Here's how the part is built. I have some questions about the finished solid (model axes, mm). A direction names the side the tool comes from. Round coordinates to 2 decimals unless told otherwise and drop trailing zeros. Order: outer loops, then holes, each group sorted by start corner. A loop starts at its lowest first (then second) coordinate and runs counter-clockwise, first axis right, second up. Notation, with made-up numbers: (-12, -34.5) -> (-2, -34.5) arc R12 cw to (-2, -23.5) -> close; hole circle Ø6 at (86.5, -16.75). An arc over 180 degrees is marked (long way). Use a Markdown table: item, result. Add a question column.
Autodesk Inventor part; units mm, degrees
ref_plane "YZ Plane" through (0, 0, 0) normal (1, 0, 0) x (0, 1, 0)
ref_plane "XZ Plane" through (0, 0, 0) normal (0, 1, 0) x (-1, 0, 0)
ref_plane "XY Plane" through (0, 0, 0) normal (0, 0, 1) x (1, 0, 0)
sketch "Sketch1" plane through (0, 0, 0) normal (0, 0, 1) x (1, 0, 0)
  line L0 (0, 0) -> (525.78, 0)
  line L1 (0, 0) -> (0, 101.6)
  line L2 (0, 101.6) -> (262.89, 253.3796)
  line L3 (262.89, 253.3796) -> (525.78, 101.6)
  line L4 (525.78, 101.6) -> (525.78, 0)
  line L5 (262.89, 246.0473) -> (6.35, 97.9338)
  line L6 (6.35, 97.9338) -> (6.35, 6.35)
  line L7 (6.35, 6.35) -> (519.43, 6.35)
  line L8 (519.43, 6.35) -> (519.43, 97.9338)
  line L9 (519.43, 97.9338) -> (262.89, 246.0473)
  point P0 (262.89, 0)
  dimension "d0" = 525.78
  dimension "d1" = 101.6
  dimension "d2" = 120
  dimension "d3" = 6.35
extrude "Extrusion1" add sketch "Sketch1" along normal blind 355.6
sketch "Sketch2" plane through (0, 0, 355.6) normal (0, 0, 1) x (1, 0, 0)
  line L0 (262.89, 246.0473) -> (519.43, 97.9338)
  line L1 (519.43, 97.9338) -> (519.43, 6.35)
  line L2 (519.43, 6.35) -> (6.35, 6.35)
  line L3 (6.35, 6.35) -> (6.35, 97.9338)
  line L4 (6.35, 97.9338) -> (262.89, 246.0473)
  line L5 (0, 0) -> (525.78, 0)
  line L6 (525.78, 0) -> (525.78, 101.6)
  line L7 (525.78, 101.6) -> (262.89, 253.3796)
  line L8 (262.89, 253.3796) -> (0, 101.6)
  line L9 (0, 101.6) -> (0, 0)
  circle A0 centre (262.89, 121.3796) radius 60
  dimension "d6" = 120
  dimension "d7" = 132
extrude "Extrusion2" add sketch "Sketch2" along normal blind 6.35 contours L0 L1 L2 L3 L4 | L9 L8 L7 L6 L5
sketch "Sketch3" plane through (0, 0, 0) normal (0, -1, 0) x (1, 0, 0)
  line L0 (0, 0) -> (525.78, 0) construction
  line L1 (525.78, 0) -> (525.78, 88.9)
  line L2 (525.78, 88.9) -> (0, 88.9) construction
  line L3 (0, 88.9) -> (0, 0) construction
  line L4 (86.36, 21.95) -> (86.36, 66.95) construction
  circle A0 centre (86.36, 44.45) radius 2.3812
  circle A1 centre (86.36, 21.95) radius 2.3812
  circle A2 centre (86.36, 66.95) radius 2.3812
  line L5 (146.36, 49.45) -> (146.36, 29.45) construction
  line L6 (156.36, 66.95) -> (156.36, 21.95) construction
  line L7 (146.36, 29.45) -> (166.36, 29.45) construction
  line L8 (166.36, 49.45) -> (146.36, 49.45) construction
  line L9 (86.36, 66.95) -> (226.36, 66.95) construction
  line L10 (226.36, 21.95) -> (86.36, 21.95) construction
  line L11 (86.36, 44.45) -> (226.36, 44.45) construction
  line L12 (166.36, 29.45) -> (166.36, 49.45) construction
  line L13 (226.36, 66.95) -> (226.36, 21.95) construction
  circle A3 centre (226.36, 66.95) radius 2.3813
  circle A4 centre (226.36, 44.45) radius 2.3813
  circle A5 centre (226.36, 21.95) radius 2.3813
  circle A6 centre (156.36, 39.45) radius 10
  line L14 (0, 0) -> (0, 361.95)
  line L15 (525.78, 0) -> (525.78, 361.95)
  line L16 (0, 0) -> (525.78, 0)
  point P0 (0, 44.45)
  point P1 (146.36, 39.45)
  point P2 (166.36, 39.45)
  point P3 (262.89, 0)
  dimension "d10" = 45
  dimension "d11" = 140
  dimension "d12" = 4.7625
  dimension "d13" = 4.7625
  dimension "d14" = 4.7625
  dimension "d15" = 4.7625
  dimension "d16" = 4.7625
  dimension "d17" = 4.7625
  dimension "d18" = 60
  dimension "d19" = 7.5
  dimension "d20" = 20
  dimension "d21" = 20
  dimension "d22" = 86.36
  dimension "d23" = 88.9
extrude "Extrusion3" cut sketch "Sketch3" against normal blind 6.35
sketch "Sketch4" plane through (0, 0, 0) normal (0, -1, 0) x (1, 0, 0)
  line L0 (71.36, 0) -> (241.36, 0)
  line L1 (241.36, 0) -> (241.36, 85)
  line L2 (241.36, 85) -> (71.36, 85)
  line L3 (71.36, 85) -> (71.36, 0)
  line L4 (0, 0) -> (525.78, 0) construction
  circle A0 centre (156.36, 39.45) radius 10 construction
  point P0 (156.36, 85)
  dimension "d26" = 170
  dimension "d27" = 85
extrude "Extrusion4" [suppressed]
properties part number "CA01" material "ABS Plastic"
(1) On a 3-axis mill with a long thin cutter (end or side, diameter ignored), from which of +Z, -Z, +X, -X, +Y, -Y can I reach the whole of each face in a straight line? I mean faces 5 (the flat face through (129.605, 176.427, 178.441)), 6 (the flat face through (6.35, 53, 175)), 7 (the cylindrical face through (165.9, 3.13, 42.45)). Say none if no direction works.
(2) If we mould it in two halves opening along X, with no side actions, what happens to faces 1 (the flat face through (259, 48, 355.6)), 2 (the flat face through (525.78, 52, 178)), 3 (the flat face through (136.42, 173.03, 175.31)), 4 (the flat face through (0, 50, 178))? For each: pulls with the +X half, pulls with the -X half, needs draft (parallel to the pull), parting line crosses it, or undercut.
(3) I want a section at B-B on y = 75. List the corners of the cut face in (x, z) for me, and give its area (3 significant figures).
(4) I want a section at D-D on x = 436.5. List the corners of the cut face in (y, z) for me, and give its area (3 significant figures).
(5) I want a section at A-A on z = 326. List the corners of the cut face in (x, y) for me.
(6) I want a section at C-C on x = 156.36. List the corners of the cut face in (y, z) for me, and give its area (3 significant figures).
(7) I'm going to push flat-ended pins straight in: P1, Ø5, axis at y = 132, z = 149.5, coming from the -X side; P2, Ø2, axis at x = 324.5, z = 56.5, coming from the +Y side; P3, Ø4, axis at x = 86.36, z = 66.95, coming from the -Y side. Where does each tip first touch, or does it pass through?
(8) Please list where these lines run through material, in increasing order: probe 1 along Z at (x, y) = (226.36, 1.75); probe 2 along X at (y, z) = (79.5, 259.5); probe 3 along Y at (x, z) = (262.89, 357.75). Write a range as from..to.
Output:
| question | item | result |
|---|---|---|
| 1 | face 5 | +Z, -Z, -X, +Y |
| 1 | face 6 | -Z |
| 1 | face 7 | -Y |
| 2 | face 1 | undercut |
| 2 | face 2 | pulls with the +X half |
| 2 | face 3 | undercut |
| 2 | face 4 | pulls with the -X half |
| 3 | outline | (0, 0) -> (6.35, 0) -> (6.35, 355.6) -> (224.83, 355.6) -> (224.83, 361.95) -> (0, 361.95) -> close; (300.95, 355.6) -> (519.43, 355.6) -> (519.43, 0) -> (525.78, 0) -> (525.78, 361.95) -> (300.95, 361.95) -> close |
| 3 | area | 7,370 mm² |
| 4 | outline | (0, 0) -> (6.35, 0) -> (6.35, 355.6) -> (145.81, 355.6) -> (145.81, 0) -> (153.15, 0) -> (153.15, 361.95) -> (0, 361.95) -> close |
| 4 | area | 5,840 mm² |
| 5 | outline | (0, 0) -> (525.78, 0) -> (525.78, 101.6) -> (262.89, 253.38) -> (0, 101.6) -> close; hole (6.35, 6.35) -> (519.43, 6.35) -> (519.43, 97.93) -> (262.89, 246.05) -> (6.35, 97.93) -> close |
| 6 | outline | (0, 0) -> (6.35, 0) -> (6.35, 29.45) -> (0, 29.45) -> close; (0, 49.45) -> (6.35, 49.45) -> (6.35, 355.6) -> (184.54, 355.6) -> (184.54, 0) -> (191.87, 0) -> (191.87, 361.95) -> (0, 361.95) -> close |
| 6 | area | 5,960 mm² |
| 7 | P1 | x = 48.32 |
| 7 | P2 | y = 218.39 |
| 7 | P3 | y = 142.97 |
| 8 | probe 1 | 0..19.57, 24.33..42.07, 46.83..64.57, 69.33..361.95 |
| 8 | probe 2 | 0..6.35, 519.43..525.78 |
| 8 | probe 3 | 0..61.38, 181.38..253.38 |
